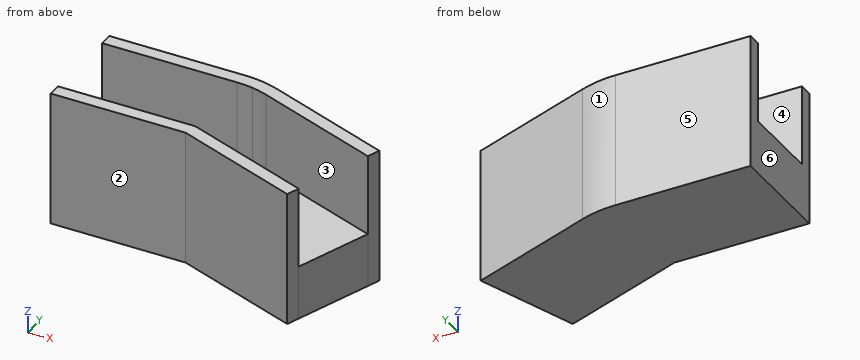
```python
from build123d import *

# Parameters (mm, degrees)
F0_W     = 50
F0_H     = 29.9999964237
F0_H_2   = 5.0000035763
F0_H_3   = 5
F1_DEPTH = 20
F2_DEPTH = 50


with BuildPart() as f1:
    # F0 (on Top) → F1 (new body)
    with BuildSketch(Plane.XY):
        with Locations((-25, 19.9999982119)):
            Rectangle(F0_W, F0_H)
        with Locations((-25, 37.4999982119)):
            Rectangle(F0_W, F0_H_2)
        with Locations((-25, 2.5)):
            Rectangle(F0_W, F0_H_3)
        with BuildLine():
            Line((0, 34.9999964237), (0, 5))
            ThreePointArc((0, 5), (0.4357787137, 4.9809734905), (0.8682408883, 4.9240387651))
            Line((0.8682408883, 4.9240387651), (6.0776855973, 34.4682678335))
            ThreePointArc((6.0776855973, 34.4682678335), (3.0504506845, 34.8668108705), (0, 34.9999964237))
        make_face()
        with BuildLine():
            Line((6.0776855973, 34.4682678335), (0.8682408883, 4.9240387651))
            ThreePointArc((0.8682408883, 4.9240387651), (1.2940952255, 4.8296291314), (1.7101007166, 4.6984631039))
            Line((1.7101007166, 4.6984631039), (11.9707037932, 32.8892383669))
            ThreePointArc((11.9707037932, 32.8892383669), (9.058665653, 33.8074004657), (6.0776855973, 34.4682678335))
        make_face()
        with BuildLine():
            Line((6.9459271067, 39.3923101205), (6.0776855973, 34.4682678335))
            ThreePointArc((6.0776855973, 34.4682678335), (9.058665653, 33.8074004657), (11.9707037932, 32.8892383669))
            Line((11.9707037932, 32.8892383669), (13.680805733, 37.5877048314))
            ThreePointArc((13.680805733, 37.5877048314), (10.3527618041, 38.6370330516), (6.9459271067, 39.3923101205))
        make_face()
        with BuildLine():
            Line((0, 40), (0, 34.9999964237))
            ThreePointArc((0, 34.9999964237), (3.0504506845, 34.8668108705), (6.0776855973, 34.4682678335))
            Line((6.0776855973, 34.4682678335), (6.9459271067, 39.3923101205))
            ThreePointArc((6.9459271067, 39.3923101205), (3.4862297099, 39.8477879237), (0, 40))
        make_face()
        with BuildLine():
            Line((0, 5), (0, 0))
            Line((0, 0), (0.8682408883, 4.9240387651))
            ThreePointArc((0.8682408883, 4.9240387651), (0.4357787137, 4.9809734905), (0, 5))
        make_face()
        with BuildLine():
            Line((0.8682408883, 4.9240387651), (0, 0))
            Line((0, 0), (1.7101007166, 4.6984631039))
            ThreePointArc((1.7101007166, 4.6984631039), (1.2940952255, 4.8296291314), (0.8682408883, 4.9240387651))
        make_face()
        Polygon((1.7101007166, 4.6984631039), (0, 0), (46.9846310393, -17.1010071663), (48.6947317559, -12.4025440624), align=None)
        Polygon((11.9707037932, 32.8892383669), (1.7101007166, 4.6984631039), (48.6947317559, -12.4025440624), (58.9553348325, 15.7882312006), align=None)
        Polygon((13.680805733, 37.5877048314), (11.9707037932, 32.8892383669), (58.9553348325, 15.7882312006), (60.6654367723, 20.4866976652), align=None)
    extrude(amount=F1_DEPTH)

    # F0 (on Top) → F2 (join)
    with BuildSketch(Plane.XY):
        with BuildLine():
            Line((6.9459271067, 39.3923101205), (6.0776855973, 34.4682678335))
            ThreePointArc((6.0776855973, 34.4682678335), (9.058665653, 33.8074004657), (11.9707037932, 32.8892383669))
            Line((11.9707037932, 32.8892383669), (13.680805733, 37.5877048314))
            ThreePointArc((13.680805733, 37.5877048314), (10.3527618041, 38.6370330516), (6.9459271067, 39.3923101205))
        make_face()
        Polygon((13.680805733, 37.5877048314), (11.9707037932, 32.8892383669), (58.9553348325, 15.7882312006), (60.6654367723, 20.4866976652), align=None)
        with BuildLine():
            Line((0, 40), (0, 34.9999964237))
            ThreePointArc((0, 34.9999964237), (3.0504506845, 34.8668108705), (6.0776855973, 34.4682678335))
            Line((6.0776855973, 34.4682678335), (6.9459271067, 39.3923101205))
            ThreePointArc((6.9459271067, 39.3923101205), (3.4862297099, 39.8477879237), (0, 40))
        make_face()
        with Locations((-25, 37.4999982119)):
            Rectangle(F0_W, F0_H_2)
        Polygon((1.7101007166, 4.6984631039), (0, 0), (46.9846310393, -17.1010071663), (48.6947317559, -12.4025440624), align=None)
        with Locations((-25, 2.5)):
            Rectangle(F0_W, F0_H_3)
        with BuildLine():
            Line((0, 5), (0, 0))
            Line((0, 0), (0.8682408883, 4.9240387651))
            ThreePointArc((0.8682408883, 4.9240387651), (0.4357787137, 4.9809734905), (0, 5))
        make_face()
        with BuildLine():
            Line((0.8682408883, 4.9240387651), (0, 0))
            Line((0, 0), (1.7101007166, 4.6984631039))
            ThreePointArc((1.7101007166, 4.6984631039), (1.2940952255, 4.8296291314), (0.8682408883, 4.9240387651))
        make_face()
    extrude(amount=F2_DEPTH)


solid = f1.part
```
Geometry: final body of the model. Coordinates: model frame, mm. Face numbers are marked on the shaded views. A direction names the side the tool comes from. Coordinates: 2 decimals unless noted, no trailing zeros. Order: outer loops, then holes, each group sorted by start corner. A loop starts at its lowest first (then second) coordinate and runs counter-clockwise, first axis right, second up. Notation, with made-up numbers: M 44,79.25 L 87,79.25 A19 ccw 87,100.25 Z; hole C -5,13.5 d6. An arc over 180 degrees is marked long. Answer in a Markdown table with one row per item. Add a question column.
Q1. Section query C-C on z = 12. Return the cut outline in (x, y), and give its area (3 significant figures).
Q2. Section query B-B on x = -5. Return the cut outline in (y, z).
Q3. Line query: L1, parallel to Y at x = -20, z = 42; L2, parallel to Z at x = -32, y = 30; L3, parallel to Y at x = -25, z = 4.5. Output: solid intervals per line, ascending.
Q4. Section query D-D on y = 30. Return the cut outline in (x, z).
Q5. Contact query for flat-ended pins moving along their axis: P1, Ø12, axis at x = -2, y = 18.5, coming from the -Z side; P2, Ø1, axis at x = 44, z = 20, coming from the -Y side; P3, Ø4, axis at x = 17.5, z = 23, coming from the +Y side; P4, Ø23.5, axis at x = -2, y = 22.5, coming from the +Z side. Output: stop coordinate, or through.
Q6. Mould query, pull axis Y, two halves, no side actions, for the marked faces 4, 5 and 6. Classes: released by +Y, released by -Y, zero draft, split by the parting line, or undercut.
Q7. Reachability of the marked faces 1, 2 and 3 from +Z, -Z, +X, -X, +Y, -Y: full face, straight path, thin tool, end or side. Return the list, or none.
Q8. Section query A-A on z = 44. Return the cut outline in (x, y).
Completed:
| question | item | result |
|---|---|---|
| 1 | outline | M -50,0 L 0,0 L 46.98,-17.1 L 60.67,20.49 L 13.68,37.59 A40 ccw 0,40 L -50,40 Z |
| 1 | area | 4,280 mm2 |
| 2 | outline | M 0,0 L 40,0 L 40,50 L 35,50 L 35,20 L 5,20 L 5,50 L 0,50 Z |
| 3 | L1 | y = 0 to 5, 35 to 40 |
| 3 | L2 | z = 0 to 20 |
| 3 | L3 | y = 0 to 40 |
| 4 | outline | M -50,0 L 34.53,0 L 34.53,50 L 19.91,50 L 19.91,20 L -50,20 Z |
| 5 | P1 | stops at z = 0 |
| 5 | P2 | stops at y = -16.2 |
| 5 | P3 | stops at y = 36.93 |
| 5 | P4 | stops at z = 20 |
| 6 | face 4 | undercut |
| 6 | face 5 | released by +Y |
| 6 | face 6 | zero draft |
| 7 | face 1 | +Z, -Z, +X, +Y |
| 7 | face 2 | +Z, -Z, -X, -Y |
| 7 | face 3 | +Z, -X |
| 8 | outline | M -50,0 L 0,0 L 46.98,-17.1 L 48.69,-12.4 L 1.71,4.7 A5 ccw 0,5 L -50,5 Z; M -50,35 L 0,35 A35 cw 11.97,32.89 L 58.96,15.79 L 60.67,20.49 L 13.68,37.59 A40 ccw 0,40 L -50,40 Z |
